Part model, mm, in its own coordinate system. A direction names the side the tool comes from. Give positions to 0.01 mm unless a question says otherwise; leave off trailing zeros. Order: outer loops, then holes, each group sorted by start corner. A loop starts at its lowest first (then second) coordinate and runs counter-clockwise, first axis right, second up.
1. Which spindle directions (+Z, -Z, +X, -X, +Y, -Y) get a long thin tool onto all of the face, cutting with end or side? Do faces 4 (the flat face through (-23, 1, -29)), 5 (the cylindrical face through (-35.077, 20.986, -53.274)), 6 (the flat face through (-19, 6, -2)). Say none if no direction does.
2. Mould opens along X. For faces 1 (the flat face through (-40, 12, -24)), 2 (the flat face through (-36, 22, 5)), 3 (the cylindrical face through (-37.998, 20.986, 2.588)) say: +X half, -X half, draft (parallel to the pull), parting line (faces both ways), or undercut.
3. Slice it at D-D on z = -44. List the corners of the cut face in (x, y), and give its area (3 significant figures).
4. Drop flat-ended pins along their axis: pin 1 Ø7.5 at (x, y) = (-15, 2.5) entering from -Z; pin 2 Ø2 at (y, z) = (16, 2.5) entering from -X; pin 3 Ø1 at (x, y) = (-15.5, 4) entering from +Z; pin 4 Ø1.2 at (x, z) = (-5, -51.5) entering from -Y. Give the stop position or say it passes through.
5. Slice it at A-A on x = -4. Give the number of separate pieces and of enclosed holes in the cut face, and give its area (3 significant figures).
6. Slice it at C-C on z = 2.5. List the corners of the cut face in (x, y), and give its area (3 significant figures).
7. Probe line 1 (Z direction, x = -4, y = 20.5); line 2 (Z direction, x = -36, y = 23.4); line 3 (Z direction, x = -33.5, y = 22.5). List the from-to ranges inside material, lowest first.
8. Slice it at B-B on y = 5. List the corners of the cut face in (x, z).
Autodesk Inventor part; units mm, degrees
ref_plane "YZ Plane" through (0, 0, 0) normal (1, 0, 0) x (0, 1, 0)
ref_plane "XZ Plane" through (0, 0, 0) normal (0, 1, 0) x (-1, 0, 0)
ref_plane "XY Plane" through (0, 0, 0) normal (0, 0, 1) x (1, 0, 0)
sketch "Sketch1" plane through (0, 0, 0) normal (0, 1, 0) x (-1, 0, 0)
  line L0 (0, 0) -> (40, 0)
  line L1 (40, 0) -> (40, -49)
  line L2 (40, -49) -> (0, -49)
  line L3 (0, -49) -> (0, 0)
  dimension "d0" = 40
  dimension "d1" = 49
extrude "Extrusion1" add sketch "Sketch1" along normal blind 24
sketch "Sketch2" plane through (0, 24, 0) normal (0, 1, 0) x (1, 0, 0)
  line L0 (0, 0) -> (0, 49)
  line L1 (0, 49) -> (-40, 49)
  line L2 (0, 0) -> (-2, 0)
  line L3 (-2, 0) -> (-2, 49)
  line L4 (-2, 49) -> (0, 49)
  line L5 (0, 49) -> (0, 0)
  line L6 (-40, 49) -> (-40, 0)
  line L7 (-40, 0) -> (-38, 0)
  line L8 (-38, 0) -> (-38, 49)
  line L9 (-38, 49) -> (-40, 49)
  line L10 (-40, 49) -> (-40, 0)
  line L11 (0, 0) -> (-40, 0)
  line L12 (-40, 0) -> (-40, 2)
  line L13 (-40, 2) -> (0, 2)
  line L14 (0, 2) -> (0, 0)
  line L15 (0, 49) -> (-40, 49)
  line L16 (-40, 49) -> (-40, 47)
  line L17 (-40, 47) -> (0, 47)
  line L18 (0, 47) -> (0, 49)
  line L19 (-2, 47) -> (-38, 47)
  line L20 (-38, 47) -> (-38, 2)
  line L21 (-38, 2) -> (-2, 2)
  line L22 (-2, 2) -> (-2, 47)
  point P0 (-38, 47)
  dimension "d4" = 2
  dimension "d5" = 2
  dimension "d6" = 2
  dimension "d7" = 2
extrude "Extrusion2" cut sketch "Sketch2" against normal blind 21.75 contours L13 L8 L17 L3
sketch "Sketch3" plane through (-40, 0, 0) normal (0, 0, 1) x (1, 0, 0)
  line L0 (0, 24) -> (40, 24)
  line L1 (0, 0) -> (40, 0)
  line L2 (0, 24) -> (8, 24)
  line L3 (8, 24) -> (8, 0)
  line L4 (8, 0) -> (0, 0)
  line L5 (0, 0) -> (0, 24)
  line L6 (0, 0) -> (0, 24)
  line L7 (40, 0) -> (40, 24)
  line L8 (0, 0) -> (40, 0)
  line L9 (40, 0) -> (40, 8)
  line L10 (40, 8) -> (0, 8)
  line L11 (0, 8) -> (0, 0)
  line L12 (38, 24) -> (2, 24)
  line L13 (40, 0) -> (32, 0)
  line L14 (32, 0) -> (32, 24)
  line L15 (32, 24) -> (40, 24)
  line L16 (40, 24) -> (40, 0)
  line L17 (8, 24) -> (32, 24)
  line L18 (32, 24) -> (32, 8)
  line L19 (32, 8) -> (8, 8)
  line L20 (8, 8) -> (8, 24)
  point P0 (8, 8)
  dimension "d10" = 8
  dimension "d11" = 8
  dimension "d12" = 8
extrude "Extrusion3" cut sketch "Sketch3" against normal blind 21 contours L0 L14 L10 L3
fillet "Fillet1" radius 5 2 edges at (-32, 8, -1) (-8, 8, -1)
sketch "Sketch4" plane through (-40, 0, 0) normal (0, 0, 1) x (1, 0, 0)
  line L0 (0, 0) -> (0, 24)
  line L1 (8, 13) -> (8, 24)
  line L2 (0, 24) -> (8, 24)
  line L3 (8, 24) -> (8, 20)
  line L4 (8, 20) -> (0, 20)
  line L5 (0, 20) -> (0, 24)
  line L6 (32, 24) -> (40, 24)
  line L7 (32, 13) -> (32, 24)
  line L8 (40, 24) -> (32, 24)
  line L9 (32, 24) -> (32, 20)
  line L10 (32, 20) -> (40, 20)
  line L11 (40, 20) -> (40, 24)
  point P0 (40, 0)
  point P1 (0, 20)
  dimension "d16" = 4
  dimension "d17" = 4
extrude "Extrusion4" add sketch "Sketch4" along normal blind 5
sketch "Sketch5" plane through (0, 0, -49) normal (0, 0, -1) x (-1, 0, 0)
  line L0 (40, 0) -> (40, 24)
  line L1 (0, 24) -> (40, 24)
  line L2 (40, 24) -> (40, 20)
  line L3 (40, 20) -> (0, 20)
  line L4 (0, 20) -> (0, 24)
  point P0 (0, 0)
  dimension "d20" = 4
extrude "Extrusion5" add sketch "Sketch5" along normal blind 5
sketch "Sketch6" plane through (-2, 24, -47) normal (-1, 0, 0) x (0, 0, 1)
  line L0 (0, 0) -> (0, -21.75)
  line L1 (0, 0) -> (45, 0)
  line L2 (0, -21.75) -> (45, -21.75)
  line L3 (45, -21.75) -> (45, 0)
  line L4 (45, 0) -> (0, 0)
  line L5 (0, 0) -> (0, -21.75)
  point P0 (47, -24)
extrude "Extrusion6" cut sketch "Sketch6" against normal blind 10
sketch "Sketch7" plane through (0, 2.25, 0) normal (0, 1, 0) x (1, 0, 0)
  line L0 (-38, 47) -> (-23, 47)
  line L1 (-23, 47) -> (-23, 36)
  line L2 (-23, 36) -> (-38, 36)
  line L3 (-38, 36) -> (-38, 47)
  line L4 (-23, 36) -> (-33, 36)
  line L5 (-33, 36) -> (-33, 23)
  line L6 (-33, 23) -> (-23, 23)
  line L7 (-23, 23) -> (-23, 36)
  line L8 (-38, 47) -> (0, 47)
  line L9 (-23, 23) -> (-18, 23)
  line L10 (-18, 23) -> (-18, 47)
  line L11 (-18, 47) -> (-23, 47)
  line L12 (-23, 47) -> (-23, 23)
  line L13 (-18, 47) -> (-7, 47)
  line L14 (-7, 47) -> (-7, 41)
  line L15 (-7, 41) -> (-18, 41)
  line L16 (-18, 41) -> (-18, 47)
  point P0 (0, 0)
  point P1 (-7, 47)
  dimension "d25" = 15
  dimension "d26" = 11
  dimension "d27" = 10
  dimension "d28" = 13
  dimension "d29" = 5
  dimension "d30" = 11
  dimension "d31" = 6
extrude "Extrusion7" cut sketch "Sketch7" against normal blind 10 contours L7 L6 L5 L2 | L8 L14 L15 L10
sketch "Sketch8" plane through (-38, 24, -47) normal (0, 0, 1) x (1, 0, 0)
  line L0 (20, -24) -> (31, -24)
  line L1 (31, -24) -> (31, -17)
  line L2 (31, -17) -> (20, -17)
  line L3 (20, -17) -> (20, -24)
  point P0 (38, -24)
  dimension "d34" = 11
  dimension "d35" = 7
extrude "Extrusion8" cut sketch "Sketch8" against normal blind 1
fillet "Fillet2" radius 1 4 edges at (-33, 1.125, -36) (-23, 1.125, -36) (-33, 1.125, -23) (-23, 1.125, -23)
sketch "Sketch9" plane through (-38, 24, -48) normal (0, 0, 1) x (1, 0, 0)
  line L0 (31, -24) -> (20, -24)
  line L1 (20, -17) -> (31, -17)
  line L2 (31, -17) -> (31, -24)
  line L3 (31, -24) -> (20, -24)
  line L4 (20, -24) -> (20, -17)
  line L5 (20, -24) -> (20, -17)
  line L6 (20, -17) -> (19, -17)
  line L7 (19, -17) -> (19, -24)
  line L8 (19, -24) -> (20, -24)
  line L9 (20, -24) -> (20, -17)
  line L10 (31, -17) -> (32, -17)
  line L11 (32, -17) -> (32, -24)
  line L12 (32, -24) -> (31, -24)
  line L13 (31, -24) -> (31, -17)
  point P0 (38, -24)
  point P1 (31, -24)
  dimension "d69" = 1
  dimension "d70" = 1
extrude "Extrusion9" add sketch "Sketch9" against normal blind 1.5
sketch "Sketch10" plane through (0, 0, 0) normal (0, -1, 0) x (1, 0, 0)
  line L0 (-8, 5) -> (0, 5)
  line L1 (0, 5) -> (-4, 5)
  line L2 (-4, 5) -> (-4, 2.5)
  line L3 (-4, 2.5) -> (0, 2.5)
  line L4 (0, 2.5) -> (0, 5)
  circle A0 centre (-4, 2.5) radius 1
  line L5 (-40, 0) -> (-40, 5)
  line L6 (-40, 5) -> (-36, 5)
  line L7 (-36, 5) -> (-36, 2.5)
  line L8 (-36, 2.5) -> (-40, 2.5)
  line L9 (-40, 2.5) -> (-40, 5)
  circle A1 centre (-36, 2.5) radius 1
  line L10 (-40, 5) -> (-40, -54)
  line L11 (-40, -54) -> (-36, -54)
  line L12 (-36, -54) -> (-36, -51.5)
  line L13 (-36, -51.5) -> (-40, -51.5)
  line L14 (-40, -51.5) -> (-40, -54)
  circle A2 centre (-36, -51.5) radius 1
  line L15 (0, -54) -> (0, -47)
  line L16 (0, -54) -> (-4, -54)
  line L17 (-4, -54) -> (-4, -51.5)
  line L18 (-4, -51.5) -> (0, -51.5)
  line L19 (0, -51.5) -> (0, -54)
  circle A3 centre (-4, -51.5) radius 1
  point P0 (0, 0)
  dimension "d41" = 4
  dimension "d42" = 2.5
  dimension "d43" = 2
  dimension "d44" = 4
  dimension "d45" = 2.5
  dimension "d46" = 2
  dimension "d49" = 4
  dimension "d50" = 2.5
  dimension "d51" = 2
  dimension "d53" = 4
  dimension "d54" = 2.5
  dimension "d55" = 2
extrude "Extrusion10" cut sketch "Sketch10" against normal blind 30 contours A0 L3 L2 | L2 L3 A0 | A1 L7 L8 | L8 L7 A1 | A2 L12 L13 | L13 L12 A2 | A3 L17 L18 | L18 L17 A3
sketch "Sketch11" plane through (-8, 20, 0) normal (0, -1, 0) x (1, 0, 0)
  circle A0 centre (4, 2.5) radius 1
  circle A1 centre (4, 2.5) radius 2
  circle A2 centre (-28, 2.5) radius 1
  circle A3 centre (-28, 2.5) radius 2
  circle A4 centre (4, -51.5) radius 1
  circle A5 centre (4, -51.5) radius 2
  circle A6 centre (-28, -51.5) radius 1
  circle A7 centre (-28, -51.5) radius 2
  point P0 (8, 0)
  dimension "d58" = 4
  dimension "d59" = 4
  dimension "d60" = 4
  dimension "d61" = 4
extrude "Extrusion11" cut sketch "Sketch11" against normal blind 2 contours A1 | A2 | A3 | A4 | A5 | A6 | A7
sketch "Sketch12" plane through (-40, 0, 0) normal (0, 0, 1) x (1, 0, 0)
  line L0 (0, 20) -> (40, 20)
  line L1 (40, 20) -> (38, 20)
  line L2 (38, 20) -> (38, 13)
  line L3 (38, 13) -> (40, 13)
  line L4 (40, 13) -> (40, 20)
  circle A0 centre (38, 13) radius 1
  point P0 (40, 0)
  dimension "d64" = 2
  dimension "d65" = 7
  dimension "d66" = 2
extrude "Extrusion12" cut sketch "Sketch12" against normal blind 5 contours A0 L3 L2 | L2 L3 A0
sketch "Sketch13" plane through (0, 20, -49) normal (0, 0, -1) x (-1, 0, 0)
  line L0 (6, -13) -> (19, -13)
  line L1 (6, -13) -> (4, -13)
  line L2 (4, -13) -> (4, -15)
  line L3 (4, -15) -> (6, -15)
  line L4 (6, -15) -> (6, -13)
  circle A0 centre (4, -15) radius 1
  point P0 (0, -20)
  dimension "d71" = 2
  dimension "d72" = 2
  dimension "d73" = 2
extrude "Extrusion13" cut sketch "Sketch13" against normal blind 3 contours A0 L3 L2 | L2 L3 A0
properties part number "encaixe1 mouse"
Data:
1. face 4: +Y, -Y
1. face 5: -Y
1. face 6: +X, +Y
2. face 1: -X half
2. face 2: draft
2. face 3: undercut
3. outline: (-40, 0) - (-18, 0) - (-18, 2.25) - (-38, 2.25) - (-38, 24) - (-40, 24) - close; (-7, 0) - (0, 0) - (0, 2.25) - (-7, 2.25) - close
3. area: 109 mm2
4. pin 1: stops at z = -49.5
4. pin 2: passes through
4. pin 3: stops at z = 0
4. pin 4: stops at y = 22
5. separate pieces: 4
5. enclosed holes: 0
5. area: 209 mm2
6. outline: (-40, 20) - (-38, 20) - (-38, 22) - (-37, 22) - (-37, 24) - (-40, 24) - close; (-35, 22) - (-34, 22) - (-34, 20) - (-32, 20) - (-32, 24) - (-35, 24) - close; (-8, 20) - (-6, 20) - (-6, 22) - (-5, 22) - (-5, 24) - (-8, 24) - close; (-3, 22) - (-2, 22) - (-2, 20) - (0, 20) - (0, 24) - (-3, 24) - close
6. area: 40.0 mm2
7. line 1: z = -54 to -53.5, -49.5 to -47, -2 to 0.5, 4.5 to 5
7. line 2: z = -54 to -52.5, -50.5 to -47, -2 to 1.5, 3.5 to 5
7. line 3: z = -54 to -47, -2 to 5
8. outline: (-40, -49) - (-19, -49) - (-19, -49.5) - (-6, -49.5) - (-6, -49) - (-5, -49) - (-5, -47) - (-7, -47) - (-7, -48) - (-18, -48) - (-18, -47) - (-38, -47) - (-38, -2) - (0, -2) - (0, 0) - (-40, 0) - close; (-3, -49) - (0, -49) - (0, -47) - (-3, -47) - close
